Build history of the part. All positions in model axes, mm. Give positions to 0.01 mm unless a question says otherwise; leave off trailing zeros. Order: outer loops, then holes, each group sorted by start corner. A loop starts at its lowest first (then second) coordinate and runs counter-clockwise, first axis right, second up. Notation, with made-up numbers: (86, 20.5) - (110, 20.5) arc R10 cw to (110, 31.5) - close; hole circle Ø2 at (28.25, -35). An arc over 180 degrees is marked (long way). Answer in a Markdown table with one row per item.
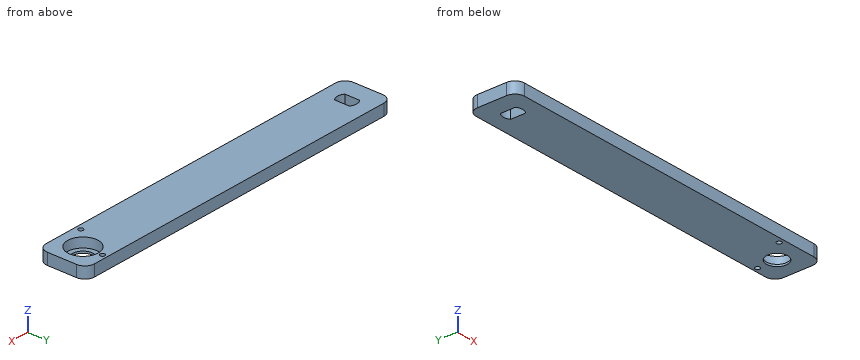
```python
from build123d import *

# Parameters (mm, degrees)
CROQUIS1_W              = 370.8
CROQUIS1_H              = 50.8
CROQUIS1_R              = 11
SALIENTE_EXTRUIR1_DEPTH = 12
REDONDEO1_R             = 10
CROQUIS4_R              = 16
CORTAR_EXTRUIR3_DEPTH   = 10
CROQUIS6_R              = 2.5
CORTAR_EXTRUIR4_DEPTH   = 347.540502683


with BuildPart() as part:
    # Croquis1 → Saliente-Extruir1 (new body)
    with BuildSketch(Plane.XY):
        with Locations((160, 0)):
            Rectangle(CROQUIS1_W, CROQUIS1_H)
        with Locations((320, 0)):
            Circle(CROQUIS1_R, mode=Mode.SUBTRACT)
        with BuildLine():
            Line((-6.28, -7.782133384), (-6.28, 7.782133384))
            ThreePointArc((-6.28, 7.782133384), (0, 10), (6.28, 7.782133384))
            Line((6.28, 7.782133384), (6.28, -7.782133384))
            ThreePointArc((6.28, -7.782133384), (0, -10), (-6.28, -7.782133384))
        make_face(mode=Mode.SUBTRACT)
    extrude(amount=SALIENTE_EXTRUIR1_DEPTH)

    # Redondeo1
    redondeo1_edges = [part.edges().sort_by_distance(p)[0] for p in [
        (-25.4, 25.4, 6),
        (345.4, 25.4, 6),
        (345.4, -25.4, 6),
        (-25.4, -25.4, 6),
    ]]
    fillet(redondeo1_edges, radius=REDONDEO1_R)

    # Croquis4 → Cortar-Extruir3 (cut)
    with BuildSketch(Plane.XY.offset(12)):
        with Locations((320, 0)):
            Circle(CROQUIS4_R)
    extrude(amount=-CORTAR_EXTRUIR3_DEPTH, mode=Mode.SUBTRACT)

    # Croquis6 → Cortar-Extruir4 (cut, through all)
    with BuildSketch(Plane.XY.offset(12)):
        with Locations((320, 20.5)):
            Circle(CROQUIS6_R)
        with Locations((360.5, 0)):
            Circle(CROQUIS6_R)
        with Locations((340, -40.5)):
            Circle(CROQUIS6_R)
        with Locations((299.5, -20)):
            Circle(CROQUIS6_R)
    extrude(amount=-CORTAR_EXTRUIR4_DEPTH, mode=Mode.SUBTRACT)


solid = part.part
```
1. Probe line 1 (X direction, y = 0, z = 1.45); line 2 (Y direction, x = 320, z = 9.75); line 3 (X direction, y = 1.5, z = 8.75). List the from-to ranges inside material, lowest first.
Check result:
| item | result |
|---|---|
| line 1 | x = -25.4 to -6.28, 6.28 to 309, 331 to 345.4 |
| line 2 | y = -25.4 to -16, 16 to 18, 23 to 25.4 |
| line 3 | x = -25.4 to -6.28, 6.28 to 304.07, 335.93 to 345.4 |
2. Cut at B-B on z = 5.75. Write the cut outline in (x, y), and give its area (3 significant figures).
Check result:
| item | result |
|---|---|
| outline | (-25.4, -15.4) arc R10 ccw to (-15.4, -25.4) - (335.4, -25.4) arc R10 ccw to (345.4, -15.4) - (345.4, 15.4) arc R10 ccw to (335.4, 25.4) - (-15.4, 25.4) arc R10 ccw to (-25.4, 15.4) - close; hole (-6.28, -7.78) arc R10 ccw to (6.28, -7.78) - (6.28, 7.78) arc R10 ccw to (-6.28, 7.78) - close; hole circle Ø5 at (299.5, -20); hole circle Ø32 at (320, 0); hole circle Ø5 at (320, 20.5) |
| area | 17,700 mm² |
3. Drop flat-ended pins along their axis: P1, Ø6, axis at y = -19, z = 8, coming from the +X side; P2, Ø2, axis at x = 306.5, y = 5, coming from the +Z side; P3, Ø20, axis at x = 320, y = 0, coming from the -Z side; P4, Ø6, axis at y = 19.5, z = 3, coming from the -X side. Give the stop position or say it passes through.
Check result:
| item | result |
|---|---|
| P1 | stops at x = 345.38 |
| P2 | stops at z = 2 |
| P3 | passes through |
| P4 | stops at x = -25.34 |
4. Cut at A-A on y = 0. Write the cut outline in (x, z).
Check result:
| item | result |
|---|---|
| outline | (-25.4, 0) - (-6.28, 0) - (-6.28, 12) - (-25.4, 12) - close; (6.28, 0) - (309, 0) - (309, 2) - (304, 2) - (304, 12) - (6.28, 12) - close; (331, 0) - (345.4, 0) - (345.4, 12) - (336, 12) - (336, 2) - (331, 2) - close |
